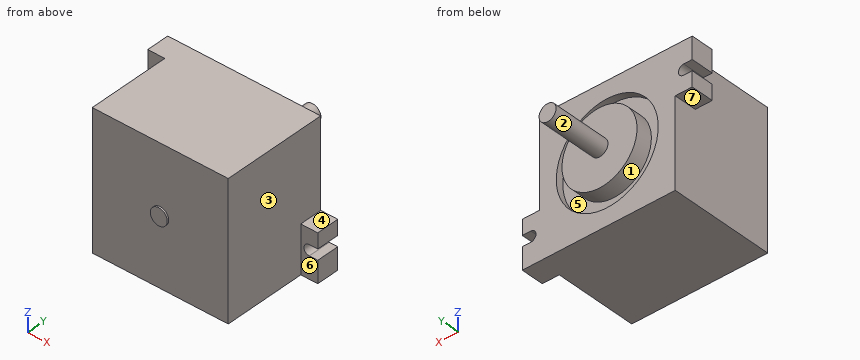
from build123d import *

# Parameters (mm, degrees)
SKETCH1_W           = 40
SKETCH1_H           = 40
BOSS_EXTRUDE1_DEPTH = 31
SKETCH2_R           = 15
CUT_EXTRUDE1_DEPTH  = 2.2
SKETCH3_R           = 11.05
BOSS_EXTRUDE2_DEPTH = 4.8
SKETCH4_R           = 2.5
BOSS_EXTRUDE3_DEPTH = 17.4
BOSS_EXTRUDE4_DEPTH = 6.7
CIRPATTERN1_COUNT   = 2
BOSS_EXTRUDE5_START = 0.5
SKETCH6_R           = 2.5
BOSS_EXTRUDE5_DEPTH = 0.5


with BuildPart() as part:
    # Sketch1 → Boss-Extrude1 (new body)
    with BuildSketch(Plane(origin=(0, 0, 0), x_dir=(1, 0, 0), z_dir=(0, 1, 0))):
        with Locations((20, 20)):
            Rectangle(SKETCH1_W, SKETCH1_H)
    extrude(amount=BOSS_EXTRUDE1_DEPTH)

    # Sketch2 → Cut-Extrude1 (cut)
    with BuildSketch(Plane(origin=(0, 31, 0), x_dir=(1, 0, 0), z_dir=(0, 1, 0))):
        with Locations(Location((20, 20, 0), (0, 0, 270))):
            Circle(SKETCH2_R)
    extrude(amount=-CUT_EXTRUDE1_DEPTH, mode=Mode.SUBTRACT)

    # Sketch3 → Boss-Extrude2 (add)
    with BuildSketch(Plane(origin=(0, 28.8, 0), x_dir=(1, 0, 0), z_dir=(0, 1, 0))):
        with Locations(Location((20, 20, 0), (0, 0, 270))):
            Circle(SKETCH3_R)
    extrude(amount=BOSS_EXTRUDE2_DEPTH)

    # Sketch4 → Boss-Extrude3 (add)
    with BuildSketch(Plane(origin=(0, 33.6, 0), x_dir=(1, 0, 0), z_dir=(0, 1, 0))):
        with Locations(Location((20, 20, 0), (0, 0, 270))):
            Circle(SKETCH4_R)
    extrude(amount=BOSS_EXTRUDE3_DEPTH)

    # Sketch5 → Boss-Extrude4 (add)
    with BuildSketch(Plane(origin=(0, 31, 0), x_dir=(1, 0, 0), z_dir=(0, 1, 0))):
        with BuildLine():
            Line((40, 40), (45, 40))
            Line((45, 40), (45, 33.55))
            Line((45, 33.55), (42.5, 33.55))
            ThreePointArc((42.5, 33.55), (40.95, 32), (42.5, 30.45))
            Line((42.5, 30.45), (45, 30.45))
            Line((45, 30.45), (45, 26))
            Line((45, 26), (40, 26))
            Line((40, 26), (40, 40))
        make_face()
    boss_extrude4 = extrude(amount=-BOSS_EXTRUDE4_DEPTH)

    # CirPattern1: Boss-Extrude4 ×2 about axis
    cirpattern1_axis = Axis((20, 0, -20), (0, 1, 0))
    for i in range(1, CIRPATTERN1_COUNT):
        add(boss_extrude4.rotate(cirpattern1_axis, i * 360 / CIRPATTERN1_COUNT))

    # Sketch6 → Boss-Extrude5 (add)
    with BuildSketch(Plane.XZ.offset(BOSS_EXTRUDE5_START)):
        with Locations(Location((20, -20, 0), (0, 0, 90))):
            Circle(SKETCH6_R)
    extrude(amount=-BOSS_EXTRUDE5_DEPTH)


solid = part.part
Check sheet for the modelled part. Datum: model origin and axes. Units: mm. Face numbers are marked on the shaded views. A direction names the side the tool comes from. Coordinates: 2 decimals unless noted, no trailing zeros. Loops run counter-clockwise (first coordinate to the right, second up) from the corner with the lowest first, then second, coordinate; pieces in that order, holes last. Notation, with made-up numbers: (36, 59) -> (72, 59) arc R16 cw to (72, 72) -> close; hole circle Ø3 at (76.5, 41.5). An arc over 180 degrees is marked (long way). Write item = value, one per line. Start each with the question number.
1. Draft check along Z on the marked faces 1, 2 and 3. Enter one of: released by +Z, released by -Z, zero draft, split by the parting line, or undercut.
2. Section check D-D on z = -20. Record the cut outline in (x, y), then the cut area to 3 significant figures.
3. Section check C-C on y = 12.5. Record the cut outline in (x, z).
4. Depth check by flat-ended pin: P1, Ø2, axis at y = 31, z = -30.5, coming from the +X side; P2, Ø12, axis at x = 13.5, z = -29.5, coming from the +Y side; P3, Ø1.5, axis at x = 23.5, z = -32, coming from the +Y side; P4, Ø12, axis at x = 36, z = -36, coming from the +Y side. Enter the tip coordinate at first touch or a pass-through.
5. Section check A-A on z = -32. Record the cut outline in (x, y), then the cut area to 3 significant figures.
6. Section check B-B on x = 15.5. Record the cut outline in (y, z), then the cut area to 3 significant figures.
7. Tool access check on the marked faces 4, 5, 6 and 7. Record the directions out of +Z, -Z, +X, -X, +Y, -Y that give a thin tool (end or side, any length) a straight path to the whole face; none if there is none.
8. Material ranges on line 1 (X direction, y = 30.1, z = -20); line 2 (Y direction, x = 13, z = -4); line 3 (Y direction, x = 33, z = -15.5), recorded low to high.
Responses:
q1.face_1 = undercut
q1.face_2 = split by the parting line
q1.face_3 = zero draft
q2.outline = (0, 0) -> (17.5, 0) -> (17.5, -0.5) -> (22.5, -0.5) -> (22.5, 0) -> (40, 0) -> (40, 31) -> (35, 31) -> (35, 28.8) -> (31.05, 28.8) -> (31.05, 33.6) -> (22.5, 33.6) -> (22.5, 51) -> (17.5, 51) -> (17.5, 33.6) -> (8.95, 33.6) -> (8.95, 28.8) -> (5, 28.8) -> (5, 31) -> (0, 31) -> close
q2.area = 1,370 mm2
q3.outline = (0, -40) -> (40, -40) -> (40, 0) -> (0, 0) -> close
q4.P1 = 45
q4.P2 = 33.6
q4.P3 = 28.8
q4.P4 = 31
q5.outline = (0, 0) -> (40, 0) -> (40, 24.3) -> (40.95, 24.3) -> (40.95, 31) -> (29, 31) -> (29, 28.8) -> (11, 28.8) -> (11, 31) -> (0, 31) -> close
q5.area = 1,210 mm2
q6.outline = (0, -40) -> (31, -40) -> (31, -34.31) -> (28.8, -34.31) -> (28.8, -30.09) -> (33.6, -30.09) -> (33.6, -9.91) -> (28.8, -9.91) -> (28.8, -5.69) -> (31, -5.69) -> (31, 0) -> (0, 0) -> close
q6.area = 1,270 mm2
q7.face_4 = +Z, +X, +Y, -Y
q7.face_5 = +Y
q7.face_6 = +Z, -Z, +X, -Y
q7.face_7 = -Z, -X, +Y, -Y
q8.line_1 = 0 to 5, 8.95 to 31.05, 35 to 40
q8.line_2 = 0 to 31
q8.line_3 = 0 to 28.8
